For this review, take the finished solid that the model builds, in its own axes (mm). A direction names the side the tool comes from. Coordinates: 2 decimals unless noted, no trailing zeros. Loops run counter-clockwise (first coordinate to the right, second up) from the corner with the lowest first, then second, coordinate; pieces in that order, holes last. Notation, with made-up numbers: (82.25, 58) -> (138.25, 58) arc R19 ccw to (138.25, 69) -> close; hole circle Ø8 at (-8.75, 85). An arc over 180 degrees is marked (long way). One line per item, written item: value.
from build123d import *

# Parameters (mm, degrees)
F0_W     = 110
F0_H     = 70
F0_R     = 2.5
F0_R_2   = 25
F1_DEPTH = 6
F2_W     = 5
F2_H     = 70
F3_DEPTH = 50
F4_W     = 77
F4_H     = 5
F5_DEPTH = 50
F7_DEPTH = 84.5
F8_SIZE  = 2
F9_SIZE  = 2


with BuildPart() as f1:
    # F0 (on Top) → F1 (new body)
    with BuildSketch(Plane.XY):
        Rectangle(F0_W, F0_H)
        with Locations((40, -12)):
            Circle(F0_R, mode=Mode.SUBTRACT)
        with Locations((-15, 0)):
            Circle(F0_R_2, mode=Mode.SUBTRACT)
        with Locations((40, 12)):
            Circle(F0_R, mode=Mode.SUBTRACT)
    extrude(amount=F1_DEPTH)

    # F2 (on face) → F3 (join)
    with BuildSketch(Plane(origin=(0, 0, 0), x_dir=(1, 0, 0), z_dir=(0, 0, -1))):
        with Locations((24.5, 0)):
            Rectangle(F2_W, F2_H)
    extrude(amount=F3_DEPTH)

    # F4 (on face) → F5 (join)
    with BuildSketch(Plane(origin=(0, 0, 0), x_dir=(1, 0, 0), z_dir=(0, 0, -1))):
        with Locations((-16.5, 32.5)):
            Rectangle(F4_W, F4_H)
        with Locations((-16.5, -32.5)):
            Rectangle(F4_W, F4_H)
    extrude(amount=F5_DEPTH)

    # F6 (on face) → F7 (cut)
    with BuildSketch(Plane.XZ.offset(35)):
        Polygon((24, -50), (-55, 0), (-55, -50), align=None)
    extrude(amount=-F7_DEPTH, mode=Mode.SUBTRACT)

    # F8
    f8_edges = [f1.edges().sort_by_distance(p)[0] for p in [
        (37.5, 12, 6),
    ]]
    chamfer(f8_edges, length=F8_SIZE)

    # F9
    f9_edges = [f1.edges().sort_by_distance(p)[0] for p in [
        (37.5, -12, 6),
    ]]
    chamfer(f9_edges, length=F9_SIZE)


solid = f1.part
1. For faces 5 (the flat face through (-43, 0, 0)), 6 (the flat face through (27, 0, -25)), 7 (the flat face through (25, 0, -50)), list the 3-axis set-ups (+Z, -Z, +X, -X, +Y, -Y) from which the entire face can be reached by the end or side of a thin tool; tool diameter is ignored.
Return value:
face 5: -Z, -X
face 6: -Z, +X, +Y, -Y
face 7: -Z, +X, -X, +Y, -Y
2. Take a section at C-C, the plane z = -23.5. Give the boundary of the cut face in (x, y), and give its area (3 significant figures).
Return value:
outline: (-17.87, -35) -> (27, -35) -> (27, 35) -> (-17.87, 35) -> (-17.87, 30) -> (22, 30) -> (22, -30) -> (-17.87, -30) -> close
area: 749 mm2
3. Take a section at D-D, the plane x = -4.5. Give the boundary of the cut face in (y, z), and give its area (3 significant figures).
Return value:
outline: (-35, -31.96) -> (-30, -31.96) -> (-30, 0) -> (-22.69, 0) -> (-22.69, 6) -> (-35, 6) -> close; (22.69, 0) -> (30, 0) -> (30, -31.96) -> (35, -31.96) -> (35, 6) -> (22.69, 6) -> close
area: 467 mm2
4. Insertion check: pin 1 Ø8.5 at (x, y) = (34, -14.5) entering from -Z; pin 2 Ø24.5 at (y, z) = (-12, -22.5) entering from -X; pin 3 Ø4 at (x, y) = (40, -12) entering from +Z; pin 4 Ø5 at (y, z) = (6, -43) entering from +X. Each pin has a flat end and moves straight along its axis. Give the tip position at first contact, or say it passes through.
Return value:
pin 1: stops at z = 0
pin 2: stops at x = 22
pin 3: passes through
pin 4: stops at x = 27
5. Take a section at A-A, the plane z = 2. Give the boundary of the cut face in (x, y), and give its area (3 significant figures).
Return value:
outline: (-55, -35) -> (55, -35) -> (55, 35) -> (-55, 35) -> close; hole circle Ø50 at (-15, 0); hole circle Ø5 at (40, -12); hole circle Ø5 at (40, 12)
area: 5,700 mm2
6. To check wall thickness, follow probe 1 along Y at (x, z) = (40, 3.25); probe 2 along Y at (x, z) = (-22.5, -17); probe 3 along Z at (x, y) = (3, 22). State the ranges of each line that lie inside material, in increasing order. Write a range as from..to.
Return value:
probe 1: y = -35..-14.5, -9.5..9.5, 14.5..35
probe 2: y = -35..-30, 30..35
probe 3: z = 0..6
7. Take a section at B-B, the plane y = -22.5. Give the boundary of the cut face in (x, z), and give its area (3 significant figures).
Return value:
outline: (-55, 0) -> (-25.9, 0) -> (-25.9, 6) -> (-55, 6) -> close; (-4.1, 0) -> (22, 0) -> (22, -48.73) -> (24, -50) -> (27, -50) -> (27, 0) -> (55, 0) -> (55, 6) -> (-4.1, 6) -> close
area: 778 mm2
8. The part is to be moulded in two halves that separate along X. For faces 1 (the cylindrical face through (42.31, 11.04, 1.97)), 2 (the flat face through (41, 0, 0)), 3 (the flat face through (55, 0, 3)), 4 (the cylindrical face through (-35, -15, 3)), say which applies: pulls with the +X half, pulls with the -X half, needs draft (parallel to the pull), parting line crosses it, or undercut.
Return value:
face 1: undercut
face 2: needs draft
face 3: pulls with the +X half
face 4: undercut
